```python
from build123d import *

# Parameters (mm, degrees)
F1_DEPTH    = 1930.4
F2_T1_DEPTH = 272.7606343602


# Not quite as in the source:
# - a fillet or chamfer that OpenCascade refuses, or shapes differently, is made with other operations: its cross-section is extruded or revolved along the edge and cut away or added


with BuildPart() as f1:
    # F0 (on Front) → F1 (new body)
    with BuildSketch(Plane.XZ):
        Polygon((0, 38.1), (0, 0), (76.2, 0), (76.2, 38.1), (50.8, 38.1), (50.8, 31.75), (25.4, 31.75), (25.4, 38.1), align=None)
    extrude(amount=F1_DEPTH)

    # F2: chamfer of 38.1 x 29.7669823699 on 1 edges, made by hand

    # F2_s2 → F2_t1 (cut)
    with BuildSketch(Plane.YZ.offset(-98.2803171801)):
        Polygon((-1900.6330176301, 0), (-1930.4, 38.1), (-1930.4, 0), align=None)
    extrude(amount=F2_T1_DEPTH, mode=Mode.SUBTRACT)


solid = f1.part
```
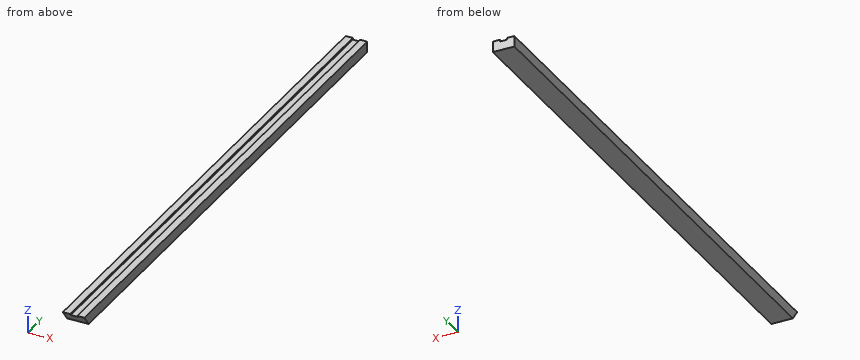
Read the model definition and answer for the solid it produces. Units are mm, in the model's axes. Round coordinates to 2 decimals unless told otherwise and drop trailing zeros. Write each loop counter-clockwise with the first axis right and the second up, starting at its lowest first coordinate (ties: lowest second). Pieces come first, ordered by that corner, then holes. Notation, with made-up numbers: (50.5, 88) - (77.5, 88) arc R24 ccw to (77.5, 127) - close; hole circle Ø2 at (-4.75, 33.25). An arc over 180 degrees is marked (long way). One line per item, written item: value.
Q1. Straight lines are drawn through the part: line 1 (X direction, y = -635, z = 33); line 2 (Z direction, x = 34.5, y = -1010); line 3 (Y direction, x = 12.5, z = 32). For each, find the intervals that lie inside material, in ascending order. Write a range as from..to.
The answers:
line 1: x = 0..25.4, 50.8..76.2
line 2: z = 0..31.75
line 3: y = -1925.63..0
Q2. This flat-tipped pin is pushed along its axis until it touches: P1, Ø7.5, axis at x = 32, y = -800.5, coming from the +Z side. Where does it stop, or does it pass through?
The answers:
P1: stops at z = 31.75
Q3. Find section A-A (y = -1699.5). Determine the outline of the cut face in (x, z).
The answers:
outline: (0, 0) - (76.2, 0) - (76.2, 38.1) - (50.8, 38.1) - (50.8, 31.75) - (25.4, 31.75) - (25.4, 38.1) - (0, 38.1) - close
